Design review of the part shown in the three views and the two pictorial views. Dimensions are in mm from the part's minimum x, y and z. A direction names the side the tool comes from. Round coordinates to 2 decimals unless told otherwise and drop trailing zeros. Write each loop counter-clockwise with the first axis right and the second up, starting at its lowest first coordinate (ties: lowest second). Pieces come first, ordered by that corner, then holes. Notation, with made-up numbers: (-23, 38) -> (-2, 38) arc R30 cw to (-2, 77) -> close; hole circle Ø2 at (57.25, 81.5). An arc over 180 degrees is marked (long way). Return JSON: item names as keys, results as strings. Group by question number.
1. Take a section at D-D, the plane y = 15.5. Write out the cut boundary in (x, z) (1 decimal), then the cut area to 3 significant figures.
2. For line 1 along Z through (x, y) = (6.65, 8.5); line 2 along Z through (x, y) = (2.5, 6.25) (1 decimal); line 3 along Y through (x, z) = (7, 9.25), list the stretches that pass through material, from the lowest coordinate up. Write a range as from..to.
3. Clearance check with flat-ended pins moving along their axes: P1, Ø2, axis at y = 4, z = 2, coming from the +X side; P2, Ø4.5, axis at y = 8.5, z = 8.5, coming from the +X side; P3, Ø3.5, axis at x = 7, y = 10.5, coming from the -Z side; P4, Ø1, axis at x = 1, y = 10, coming from the +Z side. State where each tip first meets the part, or that it passes through.
4. Mouldability with a two-part tool opening along Y and no side actions: class the marked faces 1, 2, 3 and 4 as pulls with the +Y half, pulls with the -Y half, needs draft (parallel to the pull), parting line crosses it, or undercut.
5. Take a section at C-C, the plane z = 6.5. Write out the cut boundary in (x, y), then the cut area to 3 significant figures.
6. Tool access review of the marked faces 5, 6 and 7: name each direction out of +Z, -Z, +X, -X, +Y, -Y from which nothing blocks a thin tool from reaching the whole face with its end or side.
7. Take a section at A-A, the plane x = 2.5. Write out the cut boundary in (y, z) (1 decimal), then the cut area to 3 significant figures.
8. Take a section at B-B, the plane y = 8.5. Write out the cut boundary in (x, z) (1 decimal).
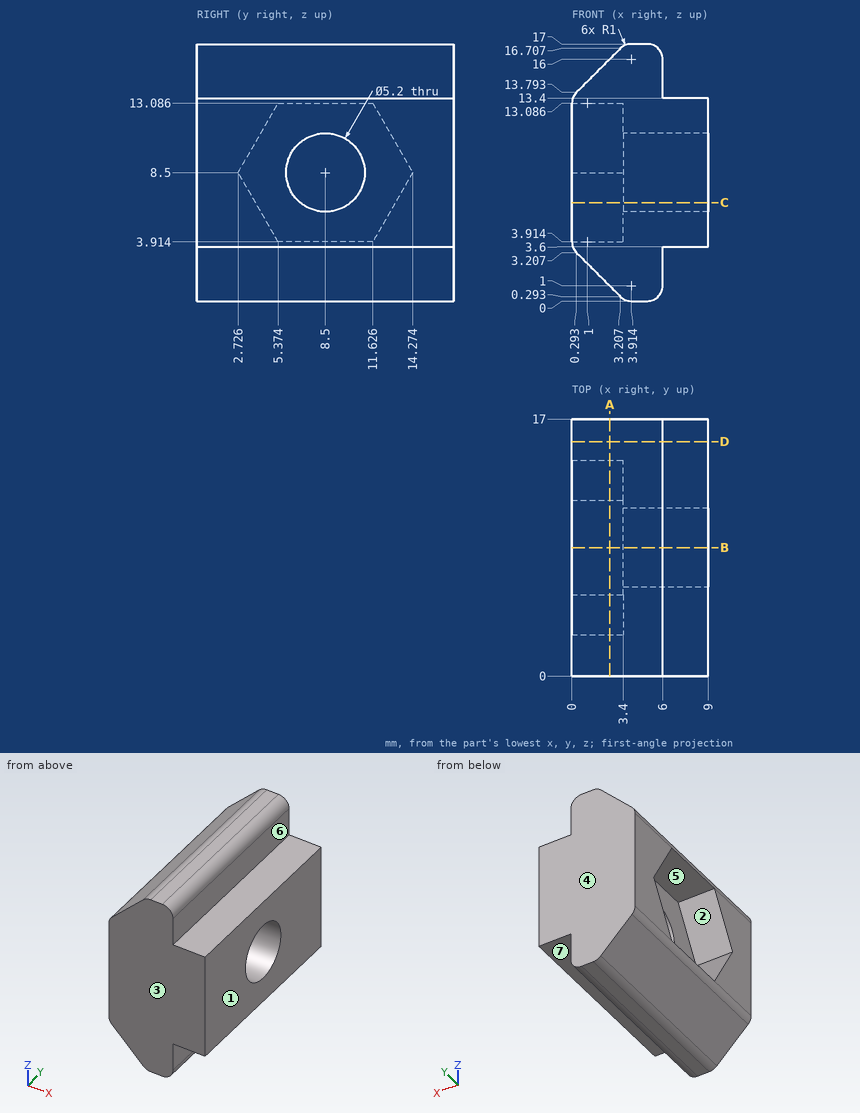
Output:
{
 "1": {"outline": "(0, 3.9) arc R1 ccw to (0.3, 3.2) -> (3.2, 0.3) arc R1 ccw to (3.9, 0) -> (5, 0) arc R1 ccw to (6, 1) -> (6, 3.6) -> (9, 3.6) -> (9, 13.4) -> (6, 13.4) -> (6, 16) arc R1 ccw to (5, 17) -> (3.9, 17) arc R1 ccw to (3.2, 16.7) -> (0.3, 13.8) arc R1 ccw to (0, 13.1) -> close", "area": "119 mm^2"},
 "2": {"line 1": "z = 3.6..5.9, 11.1..13.4", "line 2": "z = 1..3.9, 13.1..16", "line 3": "y = 0..6.01, 10.99..17"},
 "3": {"P1": "stops at x = 6", "P2": "passes through", "P3": "stops at z = 0.03", "P4": "stops at z = 15"},
 "4": {"face 1": "needs draft", "face 2": "undercut", "face 3": "pulls with the -Y half", "face 4": "pulls with the +Y half"},
 "5": {"outline": "(0, 0) -> (9, 0) -> (9, 6.84) -> (3.4, 6.84) -> (3.4, 3.88) -> (0, 3.88) -> close; (0, 13.12) -> (3.4, 13.12) -> (3.4, 10.16) -> (9, 10.16) -> (9, 17) -> (0, 17) -> close", "area": "103 mm^2"},
 "6": {"face 5": "-X", "face 6": "+Z, +X, +Y, -Y", "face 7": "-Z, +X, +Y, -Y"},
 "7": {"outline": "(0, 1) -> (17, 1) -> (17, 16) -> (0, 16) -> close; hole (2.7, 8.5) -> (5.4, 3.9) -> (11.6, 3.9) -> (14.3, 8.5) -> (11.6, 13.1) -> (5.4, 13.1) -> close", "area": "173 mm^2"},
 "8": {"outline": "(0, 3.9) arc R1 ccw to (0.3, 3.2) -> (3.2, 0.3) arc R1 ccw to (3.9, 0) -> (5, 0) arc R1 ccw to (6, 1) -> (6, 3.6) -> (9, 3.6) -> (9, 5.9) -> (3.4, 5.9) -> (3.4, 3.9) -> close; (0, 13.1) -> (3.4, 13.1) -> (3.4, 11.1) -> (9, 11.1) -> (9, 13.4) -> (6, 13.4) -> (6, 16) arc R1 ccw to (5, 17) -> (3.9, 17) arc R1 ccw to (3.2, 16.7) -> (0.3, 13.8) arc R1 ccw to start"}
}
